Geometry check sheet. Reference: drawing and pictorial views, mm from the part's lowest x, y, z. A direction names the side the tool comes from. Coordinates: 2 decimals unless noted, no trailing zeros. Loops run counter-clockwise (first coordinate to the right, second up) from the corner with the lowest first, then second, coordinate; pieces in that order, holes last. Notation, with made-up numbers: (73.5, -39) -> (114.5, -39) arc R19 ccw to (114.5, -33) -> close; hole circle Ø8 at (-6, 6). An arc over 180 degrees is marked (long way). Answer as a JSON object with one key per item and string values.
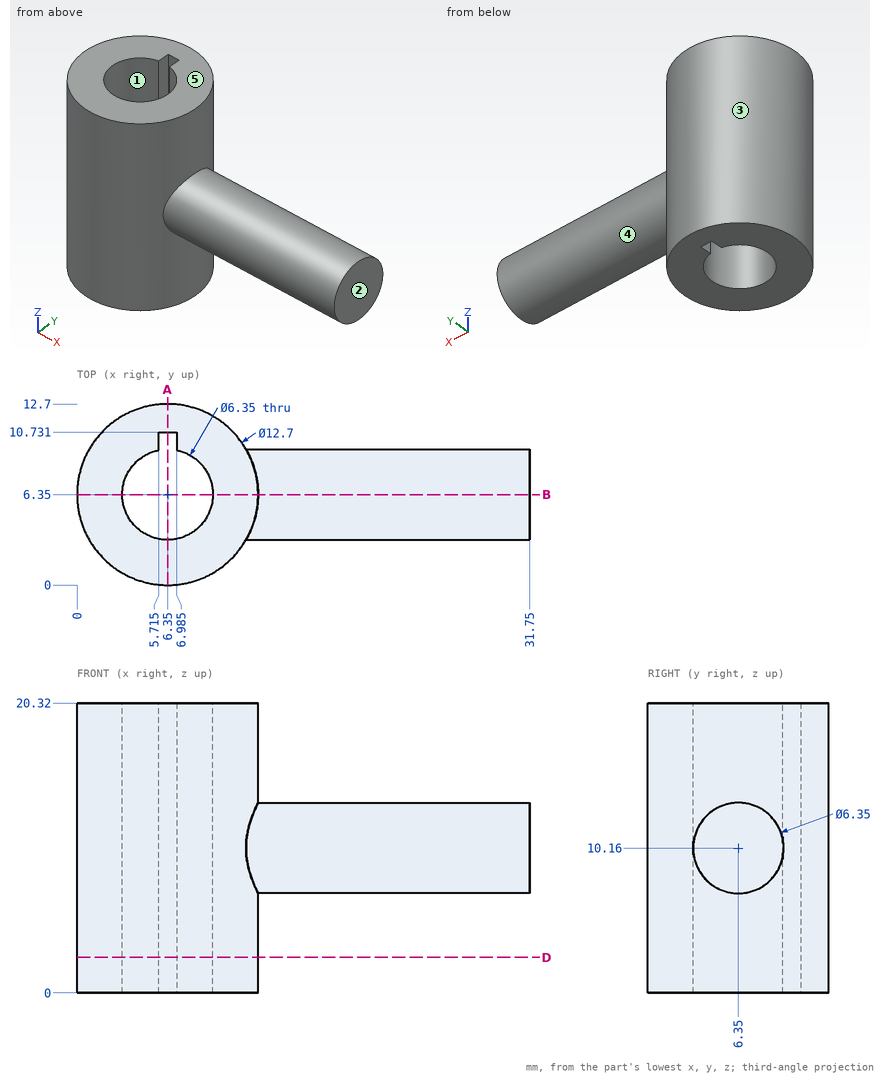
1. Section check D-D, the plane z = 2.5. Record the boundary of the cut face in (x, y) (3 decimals).
Evaluation:
{"outline": "circle Ø12.7 at (6.35, 6.35); hole (5.715, 9.461) arc R3.175 ccw (long way) to (6.985, 9.461) -> (6.985, 10.731) -> (5.715, 10.731) -> close"}
2. Tool access check on the marked faces 4 and 5. Record the directions out of +Z, -Z, +X, -X, +Y, -Y that give a thin tool (end or side, any length) a straight path to the whole face; none if there is none.
Evaluation:
{"face 4": "+X", "face 5": "+Z, +X, -X, +Y, -Y"}
3. Mould release check, pull along Y, two halves, no side actions. Record for the marked faces 1, 2 and 3: released by +Y, released by -Y, zero draft, split by the parting line, or undercut.
Evaluation:
{"face 1": "undercut", "face 2": "zero draft", "face 3": "split by the parting line"}
4. Section check A-A, the plane x = 6.35. Record the boundary of the cut face in (y, z) (3 decimals), then the cut area to 3 significant figures.
Evaluation:
{"outline": "(0, 0) -> (3.175, 0) -> (3.175, 20.32) -> (0, 20.32) -> close; (10.731, 0) -> (12.7, 0) -> (12.7, 20.32) -> (10.731, 20.32) -> close", "area": "105 mm^2"}
5. Depth check by flat-ended pin: P1, Ø1, axis at y = 10, z = 9, coming from the +X side; P2, Ø3, axis at x = 8.5, z = 10, coming from the +Y side; P3, Ø1, axis at y = 10, z = 8.5, coming from the -X side. Enter the tip coordinate at first touch or a pass-through.
Evaluation:
{"P1": "stops at x = 11.86", "P2": "stops at y = 12.67", "P3": "stops at x = 0.84"}
6. Section check B-B, the plane y = 6.35. Record the boundary of the cut face in (x, z) (3 decimals).
Evaluation:
{"outline": "(0, 0) -> (3.175, 0) -> (3.175, 20.32) -> (0, 20.32) -> close; (9.525, 0) -> (12.7, 0) -> (12.7, 6.985) -> (31.75, 6.985) -> (31.75, 13.335) -> (12.7, 13.335) -> (12.7, 20.32) -> (9.525, 20.32) -> close"}
7. Thickness scan on probe 1 along Y at (x, z) = (6.35, 11.5) (3 decimals); probe 2 along Y at (x, z) = (5.5, 12.25); probe 3 along Z at (x, y) = (22.5, 6.5). Record the ranges inside material, lowest first. Write a range as from..to.
Evaluation:
{"probe 1": "y = 0..3.175, 10.731..12.7", "probe 2": "y = 0.06..3.29, 9.41..12.64", "probe 3": "z = 6.99..13.33"}
